Could you check a few things on this model? Use its own coordinates, in mm. Coordinates: 2 decimals unless noted, no trailing zeros. Write each loop counter-clockwise with the first axis right and the second up, starting at its lowest first coordinate (ties: lowest second). Pieces come first, ordered by that corner, then holes.
```python
from build123d import *

# Parameters (mm, degrees)
F1_DEPTH = 19.05
F2_DEPTH = 12.7
F3_SIZE  = 5.08
F4_R     = 5.08


with BuildPart() as f1:
    # F0 (on Top) → F1 (new body)
    with BuildSketch(Plane.XY):
        Polygon((1.9531995618, -3.6446304457), (0, -3.6446304457), (0, -16.6841130704), (8.9412089437, -16.6841130704), (9.1255623847, -8.3420565352), (4.5166932978, -3.6446304457), align=None)
    extrude(amount=F1_DEPTH)

    # F0 (on Top) → F2 (join)
    with BuildSketch(Plane.XY):
        Polygon((1.9531995618, -3.6446304457), (0, -3.6446304457), (0, -16.6841130704), (8.9412089437, -16.6841130704), (9.1255623847, -8.3420565352), (4.5166932978, -3.6446304457), align=None)
    extrude(amount=F2_DEPTH)

    # F3
    f3_edges = [f1.edges().sort_by_distance(p)[0] for p in [
        (4.470604, -16.684113, 19.05),
    ]]
    chamfer(f3_edges, length=F3_SIZE)

    # F4
    f4_edges = [f1.edges().sort_by_distance(p)[0] for p in [
        (4.526737, -11.604113, 19.05),
        (4.470604, -16.684113, 13.97),
        (2.258347, -3.64463, 19.05),
    ]]
    fillet(f4_edges, radius=F4_R)


solid = f1.part
```
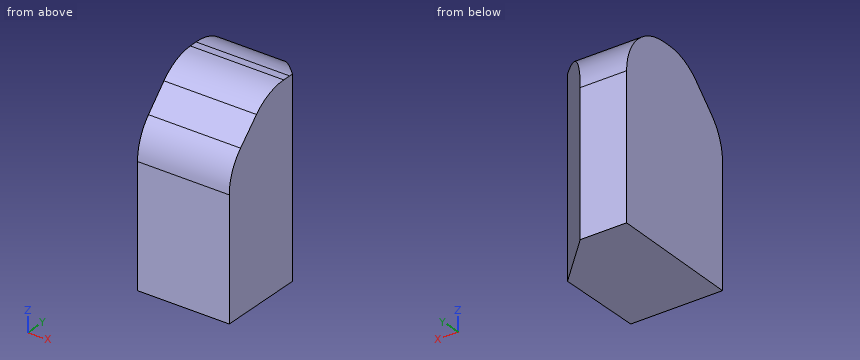
1. I want a section at A-A on x = 2.25. Please give me the cut outline in (y, z).
Verdict:
outline: (-16.68, 0) - (-3.64, 0) - (-3.64, 13.97) arc R5.08 ccw to (-8.72, 19.05) - (-9.5, 19.05) arc R5.08 ccw to (-13.09, 17.56) - (-15.2, 15.46) arc R5.08 ccw to (-16.68, 11.87) - close
2. For pin 1 (3 mm diameter, centred on x = 7.5, y = -12, fed in from +Z), with a flat end and sliding along its axis, tell me the tip position at first contact or that it passes through.
Verdict:
pin 1: stops at z = 18.95
3. I want a section at C-C on y = -11. Please give me the cut outline in (x, z), plus the area to 3 significant figures.
Verdict:
outline: (0, 0) - (9.07, 0) - (9.07, 18.82) - (0, 18.82) - close
area: 171 mm2
4. Please list where these lines run through material, in increasing order: line 1 along X through (y, z) = (-15.25, 11.5); line 2 along Y through (x, z) = (4.5, 18.25); line 3 along Y through (x, z) = (5, 16.25).
Verdict:
line 1: x = 0 to 8.97
line 2: y = -12.24 to -5.99
line 3: y = -14.4 to -4.19
5. I want a section at D-D on x = 6. Please give me the cut outline in (y, z).
Verdict:
outline: (-16.68, 0) - (-5.16, 0) - (-5.16, 17.59) arc R5.08 ccw to (-8.72, 19.05) - (-9.5, 19.05) arc R5.08 ccw to (-13.09, 17.56) - (-15.2, 15.46) arc R5.08 ccw to (-16.68, 11.87) - close
6. I want a section at B-B on z = 6.25. Please give me the cut outline in (x, y), plus the area to 3 significant figures.
Verdict:
outline: (0, -16.68) - (8.94, -16.68) - (9.13, -8.34) - (4.52, -3.64) - (0, -3.64) - close
area: 107 mm2
